```python
from build123d import *

# Parameters (mm, degrees)
F0_W     = 3
F0_H     = 3
F0_W_2   = 32
F0_H_2   = 32
F1_DEPTH = 7.5
F2_R     = 2
F3_DEPTH = 3.001
F4_R     = 2
F5_DEPTH = 35.001


with BuildPart() as f1:
    # F0 (on Front) → F1 (new body, symmetric)
    with BuildSketch(Plane.XZ):
        with Locations((-1.5, -1.5)):
            Rectangle(F0_W, F0_H)
        with Locations((16, -1.5)):
            Rectangle(F0_W_2, F0_H)
        with Locations((-1.5, -19)):
            Rectangle(F0_W, F0_H_2)
    extrude(amount=F1_DEPTH, both=True)

    # F2 (on face) → F3 (cut, through all)
    with BuildSketch(Plane.YZ):
        with Locations((0, -20)):
            Circle(F2_R)
    extrude(amount=-F3_DEPTH, mode=Mode.SUBTRACT)

    # F4 (on face) → F5 (cut, through all)
    with BuildSketch(Plane.XY):
        with Locations((17, 0)):
            Circle(F4_R)
    extrude(amount=-F5_DEPTH, mode=Mode.SUBTRACT)


solid = f1.part
```
Here's how the part is built. I have some questions about the finished solid (model axes, mm). A direction names the side the tool comes from. Coordinates: 2 decimals unless noted, no trailing zeros. Loops run counter-clockwise (first coordinate to the right, second up) from the corner with the lowest first, then second, coordinate; pieces in that order, holes last. Notation, with made-up numbers: (-11, 34.25) - (32, 34.25) arc R11 ccw to (32, 38.25) - close; hole circle Ø11 at (69.5, 82.25). An arc over 180 degrees is marked (long way). Return JSON: item names as keys, results as strings. Group by question number.
Item 1: I need wall thicknesses on line 1 (Z direction, x = -1.35, y = 0); line 2 (Y direction, x = 17, z = -2.25); line 3 (Z direction, x = 20, y = -0.75). Which ranges of each line are inside material? Lowest first, please. Write a range as from..to.
Item 2: Will these pins go through, and if not, where does the flat tip stop? P1, Ø1, axis at x = 19.5, y = -6, coming from the +Z side; P2, Ø3, axis at y = 4, z = -5, coming from the +X side; P3, Ø4, axis at x = 24, z = -5.5, coming from the -Y side.
Item 3: If we section it at D-D on x = 5: Write out the boundary of the cut face in (y, z).
Item 4: If we section it at A-A on x = 17: Write out the boundary of the cut face in (y, z), and give its area (3 significant figures).
Item 5: We'd pull the mould along Y, two halves only. Please class faces 3 (the face through (-1, -7.5, -10)), 4 (the face through (15.4, -1.2, -1.5)), 5 (the face through (16, -2, -3)), 6 (the face through (-1, 0, -18)): +Y half, -Y half, draft (parallel to the pull), parting line (faces both ways), or undercut.
Item 6: On a 3-axis mill with a long thin cutter (end or side, diameter ignored), from which of +Z, -Z, +X, -X, +Y, -Y can I reach the whole of each face in a straight line? I mean faces 1 (the face through (14.7, -0.1, 0)), 2 (the face through (0, -3, -19)). Say none if no direction works.
Item 7: If we section it at B-B on z = -20: Write out the boundary of the cut face in (x, y).
Item 8: If we section it at C-C on y = -1.5: Write out the boundary of the cut face in (x, z).
Calculated:
{
 "1": {"line 1": "z = -35..-22, -18..0", "line 2": "y = -7.5..-2, 2..7.5", "line 3": "z = -3..0"},
 "2": {"P1": "stops at z = 0", "P2": "stops at x = 0", "P3": "passes through"},
 "3": {"outline": "(-7.5, -3) - (7.5, -3) - (7.5, 0) - (-7.5, 0) - close"},
 "4": {"outline": "(-7.5, -3) - (-2, -3) - (-2, 0) - (-7.5, 0) - close; (2, -3) - (7.5, -3) - (7.5, 0) - (2, 0) - close", "area": "33.0 mm^2"},
 "5": {"face 3": "-Y half", "face 4": "undercut", "face 5": "draft", "face 6": "undercut"},
 "6": {"face 1": "+Z, +X, -X, +Y, -Y", "face 2": "-Z, +X, +Y, -Y"},
 "7": {"outline": "(-3, -7.5) - (0, -7.5) - (0, -2) - (-3, -2) - close; (-3, 2) - (0, 2) - (0, 7.5) - (-3, 7.5) - close"},
 "8": {"outline": "(-3, -35) - (0, -35) - (0, -21.32) - (-3, -21.32) - close; (-3, -18.68) - (0, -18.68) - (0, -3) - (15.68, -3) - (15.68, 0) - (-3, 0) - close; (18.32, -3) - (32, -3) - (32, 0) - (18.32, 0) - close"}
}
